from build123d import *

# Parameters (mm, degrees)
SCHIZZO1_W                   = 50
SCHIZZO1_H                   = 50
ESTRUSIONE_ESTRUSIONE1_DEPTH = 3
RACCORDO1_R                  = 5
SCHIZZO2_R                   = 7.5
ESTRUSIONE_ESTRUSIONE2_DEPTH = 15
SCHIZZO3_R                   = 0.75
TAGLIO_ESTRUSIONE1_DEPTH     = 50.737621267


with BuildPart() as part:
    # Schizzo1 → Estrusione-Estrusione1 (new body)
    with BuildSketch(Plane(origin=(0, 0, 0), x_dir=(1, 0, 0), z_dir=(0, 1, 0))):
        with Locations((9.19152509, -6.317256925)):
            Rectangle(SCHIZZO1_W, SCHIZZO1_H)
    extrude(amount=ESTRUSIONE_ESTRUSIONE1_DEPTH)

    # Raccordo1
    raccordo1_edges = [part.edges().sort_by_distance(p)[0] for p in [
        (-15.80847491, 1.5, -18.682743075),
        (34.19152509, 1.5, -18.682743075),
        (34.19152509, 1.5, 31.317256925),
        (-15.80847491, 1.5, 31.317256925),
    ]]
    fillet(raccordo1_edges, radius=RACCORDO1_R)

    # Schizzo2 → Estrusione-Estrusione2 (add)
    with BuildSketch(Plane(origin=(0, 3, 0), x_dir=(1, 0, 0), z_dir=(0, 1, 0))):
        with Locations(Location((9.19152509, -6.317256925, 0), (0, 0, 270))):
            Circle(SCHIZZO2_R)
    extrude(amount=ESTRUSIONE_ESTRUSIONE2_DEPTH)

    # Schizzo3 → Taglio-Estrusione1 (cut, through all)
    with BuildSketch(Plane(origin=(0, 18, 0), x_dir=(1, 0, 0), z_dir=(0, 1, 0))):
        with Locations(Location((9.19152509, -6.317256925, 0), (0, 0, 270))):
            Circle(SCHIZZO3_R)
    extrude(amount=-TAGLIO_ESTRUSIONE1_DEPTH, mode=Mode.SUBTRACT)


solid = part.part
Can you work these out from the model? Positions are in its coordinate system, mm. A direction names the side the tool comes from. Give positions to 0.01 mm unless a question says otherwise; leave off trailing zeros. Loops run counter-clockwise (first coordinate to the right, second up) from the corner with the lowest first, then second, coordinate; pieces in that order, holes last. Notation, with made-up numbers: (89, -36.75) - (138, -36.75) arc R14 cw to (138, -20.75) - close; hole circle Ø9 at (58, -13). An arc over 180 degrees is marked (long way). One line per item, written item: value.
(1) If we section it at D-D, the plane z = 17.5: List the corners of the cut face in (x, y) for me.
Verdict:
outline: (-15.81, 0) - (34.19, 0) - (34.19, 3) - (-15.81, 3) - close
(2) On a 3-axis mill with a long thin cutter (end or side, diameter ignored), from which of +Z, -Z, +X, -X, +Y, -Y can I reach the whole of each face in a straight line? I mean faces 1 (the face through (9, 18, 8)), 2 (the face through (11.444, 10.395, 13.471)). Say none if no direction works.
Verdict:
face 1: +Z, -Z, +X, -X, +Y
face 2: +Y
(3) I'm going to push flat-ended pins straight in: pin 1 (5 mm diameter, centred on y = 7, z = 0.5, fed in from -X) (3 decimals); pin 2 (6 mm diameter, centred on x = 5.5, y = 13.5, fed in from -Z); pin 3 (5 mm diameter, centred on x = -7, z = 12, fed in from +Y); pin 4 (5 mm diameter, centred on y = 9, z = -6, fed in from -X). Where does each tip first touch, or does it pass through?
Verdict:
pin 1: x = 2.465
pin 2: z = -1.15
pin 3: y = 3
pin 4: through
(4) If we section it at C-C, the plane y = 15.25: List the corners of the cut face in (x, z) for me, plus the area to 3 significant figures.
Verdict:
outline: circle Ø15 at (9.19, 6.32); hole circle Ø1.5 at (9.19, 6.32)
area: 175 mm^2
(5) If we section it at B-B, the plane x = 11: List the corners of the cut face in (y, z) for me.
Verdict:
outline: (0, -18.68) - (3, -18.68) - (3, -0.96) - (18, -0.96) - (18, 13.6) - (3, 13.6) - (3, 31.32) - (0, 31.32) - close
(6) I need wall thicknesses on line 1 along Y through (x, z) = (30, -2.5); line 2 along X through (y, z) = (10.5, 2); line 3 along Z through (x, y) = (7, 15.5). Which ranges of each line are inside material? Lowest first, please.
Verdict:
line 1: 0 to 3
line 2: 3.06 to 15.32
line 3: -0.86 to 13.49
(7) If we section it at A-A, the plane z = 3: List the corners of the cut face in (x, y) for me, plus the area to 3 significant figures.
Verdict:
outline: (-15.81, 0) - (34.19, 0) - (34.19, 3) - (15.92, 3) - (15.92, 18) - (2.47, 18) - (2.47, 3) - (-15.81, 3) - close
area: 352 mm^2
